Can you work these out from the model? Positions are in its coordinate system, mm. A direction names the side the tool comes from. Round coordinates to 2 decimals unless told otherwise and drop trailing zeros. Order: outer loops, then holes, each group sorted by start corner. A loop starts at its lowest first (then second) coordinate and runs counter-clockwise, first axis right, second up. Notation, with made-up numbers: (36, -9) -> (47, -9) arc R25 cw to (47, 5) -> close; hole circle Ø4 at (-16.5, -8). An arc over 180 degrees is marked (long way). One line per item, written item: value.
```python
from build123d import *

# Parameters (mm, degrees)
F1_DEPTH = 15
F2_DEPTH = 10
F3_W     = 2.5
F3_H     = 65
F4_DEPTH = 7.5


with BuildPart() as f1:
    # F0 (on Top) → F1 (new body)
    with BuildSketch(Plane.XY):
        Polygon((-34.4940570078, 34.1372138634), (-49.4940570078, 34.1372138634), (-49.4940570078, -30.8627861366), (20.7059429922, -30.8627861366), (20.7059429922, 34.1372138634), (5.7059429922, 34.1372138634), (5.7059429922, -15.8627861366), (-34.4940570078, -15.8627861366), align=None)
    extrude(amount=F1_DEPTH)

    # F0 (on Top) → F2 (join)
    with BuildSketch(Plane.XY):
        Polygon((-34.4940570078, 34.1372138634), (-49.4940570078, 34.1372138634), (-49.4940570078, -30.8627861366), (20.7059429922, -30.8627861366), (20.7059429922, 34.1372138634), (5.7059429922, 34.1372138634), (5.7059429922, -15.8627861366), (-34.4940570078, -15.8627861366), align=None)
        with BuildLine():
            Line((-21.8940570078, 34.1372138634), (-34.4940570078, 34.1372138634))
            Line((-34.4940570078, 34.1372138634), (-34.4940570078, -15.8627861366))
            Line((-34.4940570078, -15.8627861366), (5.7059429922, -15.8627861366))
            Line((5.7059429922, -15.8627861366), (5.7059429922, 34.1372138634))
            Line((5.7059429922, 34.1372138634), (-6.8940570078, 34.1372138634))
            Line((-6.8940570078, 34.1372138634), (-6.8940570078, 0))
            ThreePointArc((-6.8940570078, 0), (-14.3940570078, -7.5), (-21.8940570078, 0))
            Line((-21.8940570078, 0), (-21.8940570078, 34.1372138634))
        make_face()
    extrude(amount=F2_DEPTH)

    # F3 (on face) → F4 (cut, symmetric)
    with BuildSketch(Plane.XY):
        with Locations((-43.2440570078, 1.6372138634)):
            Rectangle(F3_W, F3_H)
        with Locations((-40.7440570078, 1.6372138634)):
            Rectangle(F3_W, F3_H)
        with BuildLine():
            Line((10.7059429922, 34.05405581), (10.7059429922, -30.8627861366))
            Line((10.7059429922, -30.8627861366), (13.2059429922, -30.8627861366))
            Line((13.2059429922, -30.8627861366), (15.7059429922, -30.8627861366))
            Line((15.7059429922, -30.8627861366), (15.7059429922, 34.05405581))
            ThreePointArc((15.7059429922, 34.05405581), (15.7055971095, 34.0956405901), (15.7045595571, 34.1372138634))
            Line((15.7045595571, 34.1372138634), (10.7073264274, 34.1372138634))
            ThreePointArc((10.7073264274, 34.1372138634), (10.7062888749, 34.0956405901), (10.7059429922, 34.05405581))
        make_face()
    extrude(amount=F4_DEPTH, both=True, mode=Mode.SUBTRACT)


solid = f1.part
```
Q1. I want a section at B-B on y = 16. List the corners of the cut face in (x, z) for me.
Answers below:
outline: (-49.49, 0) -> (-44.49, 0) -> (-44.49, 7.5) -> (-39.49, 7.5) -> (-39.49, 0) -> (-21.89, 0) -> (-21.89, 10) -> (-34.49, 10) -> (-34.49, 15) -> (-49.49, 15) -> close; (-6.89, 0) -> (10.71, 0) -> (10.71, 7.5) -> (15.71, 7.5) -> (15.71, 0) -> (20.71, 0) -> (20.71, 15) -> (5.71, 15) -> (5.71, 10) -> (-6.89, 10) -> close
Q2. We'd pull the mould along X, two halves only. Please class faces 4 (the face through (-20.3, -5.1, 0)), 5 (the face through (20.706, 1, 7)), 6 (the face through (-42, 2, 7.5)): released by +X, released by -X, zero draft, split by the parting line, or undercut.
Answers below:
face 4: zero draft
face 5: released by +X
face 6: undercut
Q3. I want a section at C-C on z = 13.75. List the corners of the cut face in (x, y) for me.
Answers below:
outline: (-49.49, -30.86) -> (20.71, -30.86) -> (20.71, 34.14) -> (5.71, 34.14) -> (5.71, -15.86) -> (-34.49, -15.86) -> (-34.49, 34.14) -> (-49.49, 34.14) -> close
Q4. On a 3-axis mill with a long thin cutter (end or side, diameter ignored), from which of +Z, -Z, +X, -X, +Y, -Y can I reach the whole of each face in a straight line? I mean faces 1 (the face through (-6.894, 17, 5)), 2 (the face through (10.706, 2, 4)), 3 (the face through (-14, -15.863, 12)). Say none if no direction works.
Answers below:
face 1: +Z, -Z, +Y
face 2: -Z, +Y, -Y
face 3: +Z, +Y
Q5. I want a section at D-D on y = -14. List the corners of the cut face in (x, z) for me, plus the area to 3 significant figures.
Answers below:
outline: (-49.49, 0) -> (-44.49, 0) -> (-44.49, 7.5) -> (-39.49, 7.5) -> (-39.49, 0) -> (10.71, 0) -> (10.71, 7.5) -> (15.71, 7.5) -> (15.71, 0) -> (20.71, 0) -> (20.71, 15) -> (5.71, 15) -> (5.71, 10) -> (-34.49, 10) -> (-34.49, 15) -> (-49.49, 15) -> close
area: 777 mm^2
Q6. I want a section at A-A on z = 5.75. List the corners of the cut face in (x, y) for me.
Answers below:
outline: (-49.49, -30.86) -> (-44.49, -30.86) -> (-44.49, 34.14) -> (-49.49, 34.14) -> close; (-39.49, -30.86) -> (10.71, -30.86) -> (10.71, 34.05) arc R2.5 cw to (10.71, 34.14) -> (-6.89, 34.14) -> (-6.89, 0) arc R7.5 cw to (-21.89, 0) -> (-21.89, 34.14) -> (-39.49, 34.14) -> close; (15.7, 34.14) arc R2.5 cw to (15.71, 34.05) -> (15.71, -30.86) -> (20.71, -30.86) -> (20.71, 34.14) -> close
Q7. Please list where these lines run through material, in increasing order: line 1 along X through (y, z) = (13, 5.5); line 2 along X through (y, z) = (-14, 3); line 3 along X through (y, z) = (28.5, 11.25).
Answers below:
line 1: -49.49 to -44.49, -39.49 to -21.89, -6.89 to 10.71, 15.71 to 20.71
line 2: -49.49 to -44.49, -39.49 to 10.71, 15.71 to 20.71
line 3: -49.49 to -34.49, 5.71 to 20.71
Q8. Will these pins go through, and if not, where does the flat tip stop? pin 1 Ø1.5 at (x, y) = (12.5, -3.5) entering from -Z; pin 2 Ø2.5 at (x, z) = (-18, 12.5) entering from +Y; pin 3 Ø12 at (x, y) = (-18.5, 3.5) entering from +Z.
Answers below:
pin 1: z = 7.5
pin 2: y = -15.86
pin 3: z = 10
